Can you work these out from the model? Positions are in its coordinate system, mm. Face numbers are marked on the shaded views. A direction names the side the tool comes from. Give positions to 0.01 mm unless a question says otherwise; leave off trailing zeros. Write each loop counter-clockwise with the first axis right and the second up, starting at its lowest first coordinate (ties: lowest second). Pieces come first, ordered by that corner, then holes.
1. If I drill on probe 1 along X at (y, z) = (325, -723.5); probe 2 along X at (y, z) = (443.5, -55); probe 3 along Z at (x, y) = (68.5, 383), over which ranges is the centre line in solid material (lowest first)?
2. Suppose I cut it at A-A (y = 919). Please give me the cut outline in (x, z), and give its area (3 significant figures).
3. Suppose I cut it at D-D (z = -524). Please give me the cut outline in (x, y).
4. Suppose I cut it at C-C (x = 940). Please give me the cut outline in (y, z).
5. Thinking about a two-plate mould opening in X: for the marked faces 1, 2, 3 and 4, which applies, pulls with the +X half, pulls with the -X half, needs draft (parallel to the pull), parting line crosses it, or undercut?
6. On a 3-axis mill with a long thin cutter (end or side, diameter ignored), from which of +Z, -Z, +X, -X, +Y, -Y can I reach the whole of each face in a straight line? I mean the marked faces 5 and 6. Say none if no direction works.
7. Suppose I cut it at B-B (y = 617). Please give me the cut outline in (x, z).
8. I'm going to push flat-ended pins straight in: pin 1 (10 mm diameter, centred on x = 298, y = 278.5, fed in from +Z); pin 2 (5 mm diameter, centred on x = 775.5, z = -703.5, fed in from +Y); pin 3 (3 mm diameter, centred on x = 939.5, z = -890.5, fed in from +Y). Where does each tip first touch, or does it pass through?
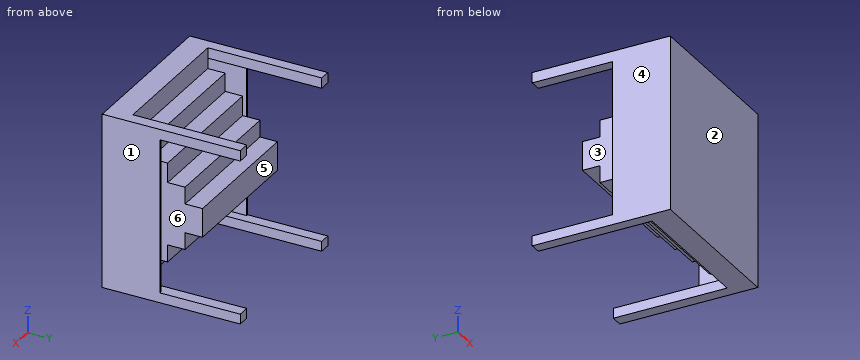
```python
from build123d import *

# Parameters (mm, degrees)
CROQUIS1_W              = 1200
CROQUIS1_H              = 1300
SALIENTE_EXTRUIR1_DEPTH = 30
CROQUIS2_W              = 83.202896363
CROQUIS2_H              = 73.82225968
CROQUIS2_W_2            = 88.769831052
CROQUIS2_H_2            = 77.533549472
SALIENTE_EXTRUIR2_DEPTH = 1000
CROQUIS3_W              = 12.688390301
CROQUIS3_H              = 1148.644190848
CROQUIS3_W_2            = 18.255324991
SALIENTE_EXTRUIR3_DEPTH = 400
CROQUIS4_W              = 1028.027272585
CROQUIS4_H              = 1300
SALIENTE_EXTRUIR4_DEPTH = 150
CROQUIS5_W              = 1028.027272585
CROQUIS5_H              = 1005.759533828
SALIENTE_EXTRUIR5_DEPTH = 130
CROQUIS6_W              = 1028.027272585
CROQUIS6_H              = 742.257958545
SALIENTE_EXTRUIR6_DEPTH = 130
CROQUIS7_W              = 1028.027272585
CROQUIS7_H              = 467.622513883
SALIENTE_EXTRUIR7_DEPTH = 130
CROQUIS8_W              = 1028.027272585
CROQUIS8_H              = 215.254807978
SALIENTE_EXTRUIR8_DEPTH = 130


with BuildPart() as part:
    # Croquis1 → Saliente-Extruir1 (new body)
    with BuildSketch(Plane(origin=(0, 0, 0), x_dir=(1, 0, 0), z_dir=(0, 1, 0))):
        with Locations((600, 650)):
            Rectangle(CROQUIS1_W, CROQUIS1_H)
    extrude(amount=SALIENTE_EXTRUIR1_DEPTH)

    # Croquis2 → Saliente-Extruir2 (add)
    with BuildSketch(Plane(origin=(0, 30, 0), x_dir=(1, 0, 0), z_dir=(0, 1, 0))):
        with Locations((41.601448182, 1263.08887016)):
            Rectangle(CROQUIS2_W, CROQUIS2_H)
        with Locations((1155.615084474, 1263.08887016)):
            Rectangle(CROQUIS2_W_2, CROQUIS2_H)
        with Locations((41.601448182, 38.766774736)):
            Rectangle(CROQUIS2_W, CROQUIS2_H_2)
        with Locations((1155.615084474, 38.766774736)):
            Rectangle(CROQUIS2_W_2, CROQUIS2_H_2)
    extrude(amount=SALIENTE_EXTRUIR2_DEPTH)

    # Croquis3 → Saliente-Extruir3 (add)
    with BuildSketch(Plane(origin=(0, 30, 0), x_dir=(1, 0, 0), z_dir=(0, 1, 0))):
        with Locations((6.344195151, 651.855644896)):
            Rectangle(CROQUIS3_W, CROQUIS3_H)
        with Locations((1190.872337505, 651.855644896)):
            Rectangle(CROQUIS3_W_2, CROQUIS3_H)
    extrude(amount=SALIENTE_EXTRUIR3_DEPTH)

    # Croquis4 → Saliente-Extruir4 (add)
    with BuildSketch(Plane(origin=(0, 30, 0), x_dir=(1, 0, 0), z_dir=(0, 1, 0))):
        with Locations((597.216532656, 650)):
            Rectangle(CROQUIS4_W, CROQUIS4_H)
    extrude(amount=SALIENTE_EXTRUIR4_DEPTH)

    # Croquis5 → Saliente-Extruir5 (add)
    with BuildSketch(Plane(origin=(0, 180, 0), x_dir=(1, 0, 0), z_dir=(0, 1, 0))):
        with Locations((597.216532656, 658.350402034)):
            Rectangle(CROQUIS5_W, CROQUIS5_H)
    extrude(amount=SALIENTE_EXTRUIR5_DEPTH)

    # Croquis6 → Saliente-Extruir6 (add)
    with BuildSketch(Plane(origin=(0, 310, 0), x_dir=(1, 0, 0), z_dir=(0, 1, 0))):
        with Locations((597.216532656, 663.917336723)):
            Rectangle(CROQUIS6_W, CROQUIS6_H)
    extrude(amount=SALIENTE_EXTRUIR6_DEPTH)

    # Croquis7 → Saliente-Extruir7 (add)
    with BuildSketch(Plane(origin=(0, 440, 0), x_dir=(1, 0, 0), z_dir=(0, 1, 0))):
        with Locations((597.216532656, 673.195561204)):
            Rectangle(CROQUIS7_W, CROQUIS7_H)
    extrude(amount=SALIENTE_EXTRUIR7_DEPTH)

    # Croquis8 → Saliente-Extruir8 (add)
    with BuildSketch(Plane(origin=(0, 570, 0), x_dir=(1, 0, 0), z_dir=(0, 1, 0))):
        with Locations((597.216532656, 673.195561205)):
            Rectangle(CROQUIS8_W, CROQUIS8_H)
    extrude(amount=SALIENTE_EXTRUIR8_DEPTH)


solid = part.part
```
Checks:
1. probe 1: x = 0 to 12.69, 83.2 to 1111.23, 1181.74 to 1200
1. probe 2: x = 0 to 83.2, 1111.23 to 1200
1. probe 3: z = -1300 to -1226.18, -77.53 to 0
2. outline: (0, -1300) - (83.2, -1300) - (83.2, -1226.18) - (0, -1226.18) - close; (0, -77.53) - (83.2, -77.53) - (83.2, 0) - (0, 0) - close; (1111.23, -1300) - (1200, -1300) - (1200, -1226.18) - (1111.23, -1226.18) - close; (1111.23, -77.53) - (1200, -77.53) - (1200, 0) - (1111.23, 0) - close
2. area: 26,000 mm2
3. outline: (0, 0) - (1200, 0) - (1200, 430) - (1181.74, 430) - (1181.74, 30) - (1111.23, 30) - (1111.23, 570) - (83.2, 570) - (83.2, 30) - (12.69, 30) - (12.69, 430) - (0, 430) - close
4. outline: (0, -1300) - (180, -1300) - (180, -1161.23) - (310, -1161.23) - (310, -1035.05) - (440, -1035.05) - (440, -907.01) - (570, -907.01) - (570, -780.82) - (700, -780.82) - (700, -565.57) - (570, -565.57) - (570, -439.38) - (440, -439.38) - (440, -292.79) - (310, -292.79) - (310, -155.47) - (180, -155.47) - (180, 0) - (0, 0) - close
5. face 1: pulls with the +X half
5. face 2: needs draft
5. face 3: undercut
5. face 4: pulls with the -X half
6. face 5: +Z, -Z, +X, -X, +Y
6. face 6: +Y
7. outline: (0, -1300) - (83.2, -1300) - (83.2, -1226.18) - (0, -1226.18) - close; (0, -77.53) - (83.2, -77.53) - (83.2, 0) - (0, 0) - close; (83.2, -780.82) - (1111.23, -780.82) - (1111.23, -565.57) - (83.2, -565.57) - close; (1111.23, -1300) - (1200, -1300) - (1200, -1226.18) - (1111.23, -1226.18) - close; (1111.23, -77.53) - (1200, -77.53) - (1200, 0) - (1111.23, 0) - close
8. pin 1: stops at z = -155.47
8. pin 2: stops at y = 700
8. pin 3: stops at y = 570
